Autodesk Inventor part; units mm, degrees
ref_plane "YZ Plane" through (0, 0, 0) normal (1, 0, 0) x (0, 1, 0)
ref_plane "XZ Plane" through (0, 0, 0) normal (0, 1, 0) x (-1, 0, 0)
ref_plane "XY Plane" through (0, 0, 0) normal (0, 0, 1) x (1, 0, 0)
sketch "Sketch1" plane through (0, 0, 0) normal (0, 1, 0) x (-1, 0, 0)
  circle A0 centre (0, 0) radius 75
  dimension "d0" = 150
extrude "Extrusion1" add sketch "Sketch1" against normal blind 100
sketch "Sketch2" plane through (0, 0, 0) normal (0, 1, 0) x (1, 0, 0)
  circle A0 centre (0, 0) radius 72
  dimension "d3" = 144
sketch "Sketch4" plane through (0, 0, 0) normal (0, 0, 1) x (1, 0, 0)
  line L0 (-75, -100) -> (75, -100)
  line L1 (0, -100) -> (23, -100)
  line L2 (75, 0) -> (-75, 0)
  line L3 (23, -100) -> (75, 0)
  line L4 (75, 0) -> (23, -100)
  line L5 (23, -100) -> (75, 0)
  line L6 (75, 0) -> (23, -100)
  line L7 (0, -100) -> (-23, -100)
  line L8 (-75, 0) -> (-23, -100)
  line L9 (75, 0) -> (75, -100)
  line L10 (23, -100) -> (75, -100)
  line L11 (0, -120) -> (0, 20)
  line L12 (75, 0) -> (72, 0)
  line L13 (72, 0) -> (20, -100)
  line L14 (20, -100) -> (0, -100)
  line L15 (0, -100) -> (0, 0)
  line L16 (0, 0) -> (72, 0)
  dimension "d5" = 23
  dimension "d10" = 23
  dimension "d14" = 3
sketch "Sketch7" plane through (0, 0, 0) normal (1, 0, 0) x (0, 1, 0)
  line L0 (0, -75) -> (0, 75)
  line L1 (0, 75) -> (-100, 75)
  line L2 (0, 75) -> (-100, 75)
  line L3 (-100, 75) -> (-100, -75)
  line L4 (-100, 75) -> (-100, 20)
  point P0 (0, 0)
  dimension "d9" = 100
sketch "Sketch11" plane through (0, -100, 0) normal (0, -1, 0) x (1, 0, 0)
  circle A0 centre (0, 0) radius 20
  circle A1 centre (0, 0) radius 23
  dimension "d11" = 40
  dimension "d12" = 46
revolve "Revolution3" cut sketch "Sketch4" angle 360 about axis through (0, -10, 0) along (0, 1, 0) contours L3 L9 L0
revolve "Revolution4" cut sketch "Sketch4" angle 360 about axis through (0, -10, 0) along (0, 1, 0) contours L11 L2 L13 L0
properties part number "cone"
Here's how the part is built. I have some questions about the finished solid (model axes, mm). Round coordinates to 2 decimals unless told otherwise and drop trailing zeros. Loops run counter-clockwise (first coordinate to the right, second up) from the corner with the lowest first, then second, coordinate; pieces in that order, holes last.
1. Suppose I cut it at D-D, the plane y = -39.5. Please give me the cut outline in (x, z), and give its area (3 significant figures).
Answers:
outline: circle Ø108.92 at (0, 0); hole circle Ø102.92 at (0, 0)
area: 998 mm2
2. Will these pins go through, and if not, where does the flat tip stop? pin 1 (6 mm diameter, centred on x = 17.5, y = -31, fed in from -Z); pin 2 (3 mm diameter, centred on y = -17, z = -57.5, fed in from -X); pin 3 (12 mm diameter, centred on y = -26, z = 49, fed in from -X).
Answers:
pin 1: stops at z = -58.07
pin 2: stops at x = -35.64
pin 3: stops at x = -45.39
3. Suppose I cut it at B-B, the plane x = 0. Please give me the cut outline in (y, z).
Answers:
outline: (-100, -23) - (0, -75) - (0, -72) - (-100, -20) - close; (-100, 20) - (0, 72) - (0, 75) - (-100, 23) - close
4. Thinking about a two-plate mould opening in Z: for faces 1 (the face through (-7.55, -71.52, 33.98)), 2 (the face through (67, 0, 28)), 3 (the face through (-8.2, -71.52, 36.91)), which applies, released by +Z, released by -Z, zero draft, split by the parting line, or undercut?
Answers:
face 1: undercut
face 2: zero draft
face 3: split by the parting line
5. Suppose I cut it at C-C, the plane y = -82. Please give me the cut outline in (x, z), and give its area (3 significant figures).
Answers:
outline: circle Ø64.72 at (0, 0); hole circle Ø58.72 at (0, 0)
area: 582 mm2
6. Suppose I cut it at A-A, the plane z = 0. Please give me the cut outline in (x, y).
Answers:
outline: (-75, 0) - (-23, -100) - (-20, -100) - (-72, 0) - close; (20, -100) - (23, -100) - (75, 0) - (72, 0) - close
7. If I drill on probe 1 along Z at (x, y) = (-48, -31); probe 2 along X at (y, z) = (-6, -53.5); probe 3 along X at (y, z) = (-53.5, 32), over which ranges is the centre line in solid material (lowest first)?
Answers:
probe 1: z = -34.1 to -28.61, 28.61 to 34.1
probe 2: x = -48.01 to -43.38, 43.38 to 48.01
probe 3: x = -34.67 to -30.46, 30.46 to 34.67
